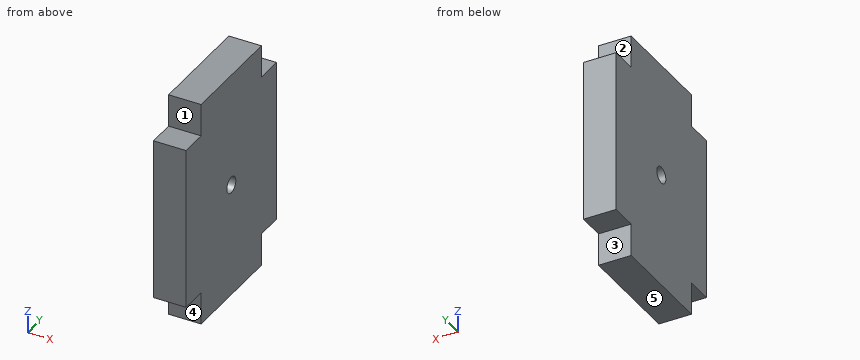
from build123d import *

# Parameters (mm, degrees)
SKICA1_W                 = 3
SKICA1_H                 = 10
SKICA1_W_2               = 15
SKICA1_H_2               = 15
P_IDAT_VYSUNUT_M1_DEPTH  = 3
SKICA2_R                 = 0.75
ODEBRAT_VYSUNUT_M1_DEPTH = 3


with BuildPart() as part:
    # Skica1 → Přidat vysunutím1 (new body)
    with BuildSketch(Plane(origin=(0, 0, 0), x_dir=(0, 0, -1), z_dir=(1, 0, 0))):
        with Locations((9, 0)):
            Rectangle(SKICA1_W, SKICA1_H)
        Rectangle(SKICA1_W_2, SKICA1_H_2)
        with Locations((-9, 0)):
            Rectangle(SKICA1_W, SKICA1_H)
    extrude(amount=P_IDAT_VYSUNUT_M1_DEPTH)

    # Skica2 → Odebrat vysunutím1 (cut)
    with BuildSketch(Plane(origin=(3, 0, 0), x_dir=(0, 0, -1), z_dir=(1, 0, 0))):
        Circle(SKICA2_R)
    extrude(amount=-ODEBRAT_VYSUNUT_M1_DEPTH, mode=Mode.SUBTRACT)


solid = part.part
Model file for the job. Use its own axes, mm. Face numbers are marked on the shaded views. A direction names the side the tool comes from. Round coordinates to 2 decimals unless told otherwise and drop trailing zeros. Loops run counter-clockwise (first coordinate to the right, second up) from the corner with the lowest first, then second, coordinate; pieces in that order, holes last. Notation, with made-up numbers: M 72,-26.75 L 99,-26.75 A18 ccw 99,-11.75 Z; hole C -6,50 d6. An arc over 180 degrees is marked long. One line per question, with ' | ' between items.
1) 3-axis set-ups, long thin cutter, end or side, ignore diameter. For the marked faces 1, 2, 3, 4 and 5: which of +Z, -Z, +X, -X, +Y, -Y reach the whole face in a straight line?
Solved:
face 1: +Z, +X, -X, -Y | face 2: +Z, +X, -X, +Y | face 3: -Z, +X, -X, +Y | face 4: -Z, +X, -X, -Y | face 5: -Z, +X, -X, +Y, -Y
2) Band-saw the part on D-D (y = 5.5). Give the cut face in (x, z), then the cut area to 3 significant figures.
Solved:
outline: M 0,-7.5 L 3,-7.5 L 3,7.5 L 0,7.5 Z | area: 45.0 mm²
3) Band-saw the part on C-C (y = 0). Give the cut face in (x, z).
Solved:
outline: M 0,-10.5 L 3,-10.5 L 3,-0.75 L 0,-0.75 Z; M 0,0.75 L 3,0.75 L 3,10.5 L 0,10.5 Z
4) Flat gauge pins, fed straight in: pin 1 (0.9 mm diameter, centred on x = 1.5, z = -9, fed in from +Y); pin 2 (1.5 mm diameter, centred on x = 2, z = -9.5, fed in from -Y); pin 3 (1.2 mm diameter, centred on y = 0, z = 0, fed in from +X); pin 4 (0.8 mm diameter, centred on x = 2, y = 7, fed in from -Z). Where does each tip first touch, or does it go through?
Solved:
pin 1: stops at y = 5 | pin 2: stops at y = -5 | pin 3: passes through | pin 4: stops at z = -7.5
5) Band-saw the part on A-A (z = 0). Give the cut face in (x, y).
Solved:
outline: M 0,-7.5 L 3,-7.5 L 3,-0.75 L 0,-0.75 Z; M 0,0.75 L 3,0.75 L 3,7.5 L 0,7.5 Z
6) Drill centre lines: line 1 along Y through (x, z) = (2.45, 0); line 2 along Z through (x, y) = (0.5, -0.25); line 3 along Z through (x, y) = (0.7, -5.25). Where is each one in solid material? Low to high.
Solved:
line 1: y = -7.5 to -0.75, 0.75 to 7.5 | line 2: z = -10.5 to -0.71, 0.71 to 10.5 | line 3: z = -7.5 to 7.5
7) Band-saw the part on B-B (x = 1). Give the cut face in (y, z).
Solved:
outline: M -7.5,-7.5 L -5,-7.5 L -5,-10.5 L 5,-10.5 L 5,-7.5 L 7.5,-7.5 L 7.5,7.5 L 5,7.5 L 5,10.5 L -5,10.5 L -5,7.5 L -7.5,7.5 Z; hole C 0,0 d1.5
